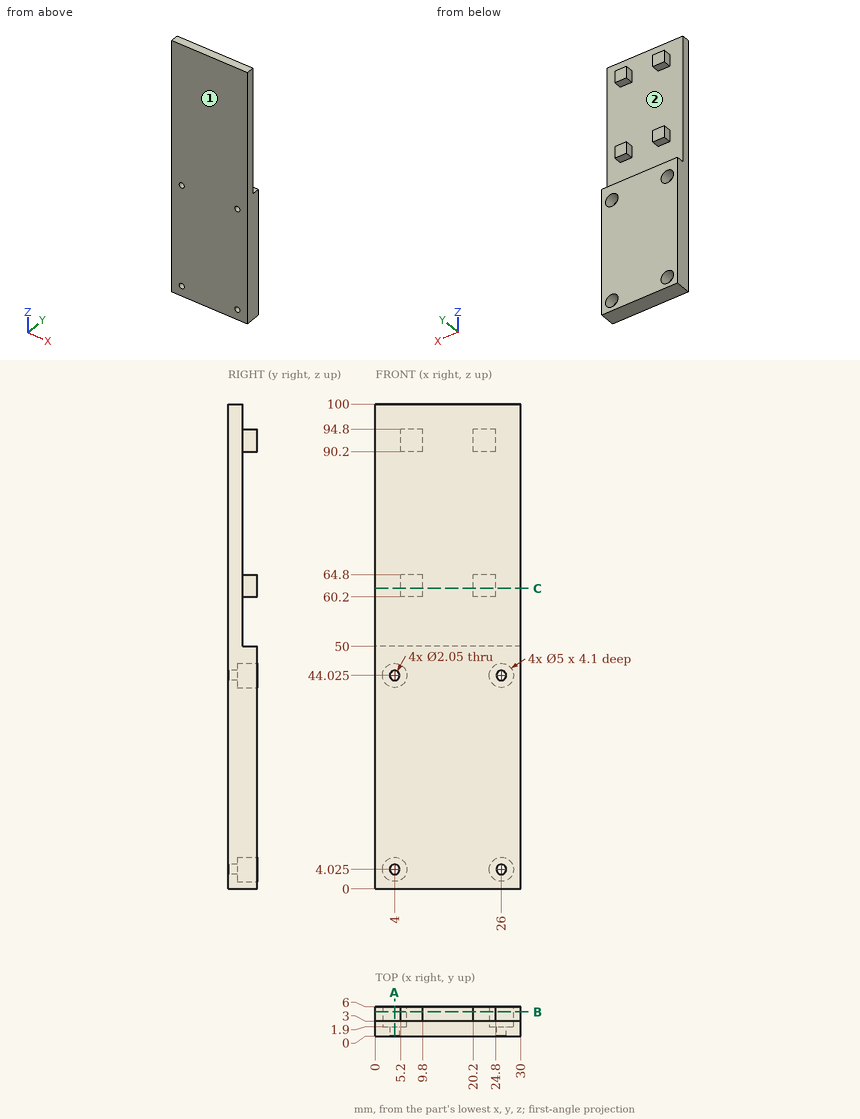
Part print with two shaded views. Sizes in mm from the minimum x, y, z corner. Give positions to 0.01 mm unless a question says otherwise; leave off trailing zeros. Order: outer loops, then holes, each group sorted by start corner. A loop starts at its lowest first (then second) coordinate and runs counter-clockwise, first axis right, second up.
1) Pin check, flat tips, straight feed: pin 1 (9 mm diameter, centred on x = 22.5, z = 74.5, fed in from +Y); pin 2 (1.5 mm diameter, centred on x = 7, y = 2.5, fed in from -Z); pin 3 (1.5 mm diameter, centred on y = 5, z = 62.5, fed in from -X); pin 4 (1.5 mm diameter, centred on x = 8.5, y = 5, fed in from +Z). Stop position of each tip, or through.
2) Mould opens along Z. For the marked faces 1 and 2 say: +Z half, -Z half, draft (parallel to the pull), parting line (faces both ways), or undercut.
3) Saw through at B-B, the plane y = 5. Count the separate pieces of the cut face and the enclosed holes in it, then the cut area to 3 significant figures.
4) Saw through at C-C, the plane z = 62. Write the cut outline in (x, y).
5) Saw through at A-A, the plane x = 4. Write the cut outline in (y, z) (3 decimals), then the cut area to 3 significant figures.
6) Wall check: probe 1 along Z at (x, y) = (4, 4.25) (3 decimals); probe 2 along Z at (x, y) = (4, 1.5); probe 3 along Y at (x, z) = (1.5, 62.5). Give the ranges that are in metal, low to high.
Computed:
1. pin 1: stops at y = 3
1. pin 2: stops at z = 0
1. pin 3: stops at x = 5.2
1. pin 4: stops at z = 94.8
2. face 1: draft
2. face 2: undercut
3. separate pieces: 5
3. enclosed holes: 4
3. area: 1,510 mm2
4. outline: (0, 0) - (30, 0) - (30, 3) - (24.8, 3) - (24.8, 6) - (20.2, 6) - (20.2, 3) - (9.8, 3) - (9.8, 6) - (5.2, 6) - (5.2, 3) - (0, 3) - close
5. outline: (0, 0) - (6, 0) - (6, 1.525) - (1.9, 1.525) - (1.9, 3) - (0, 3) - close; (0, 5.05) - (1.9, 5.05) - (1.9, 6.525) - (6, 6.525) - (6, 41.525) - (1.9, 41.525) - (1.9, 43) - (0, 43) - close; (0, 45.05) - (1.9, 45.05) - (1.9, 46.525) - (6, 46.525) - (6, 50) - (3, 50) - (3, 100) - (0, 100) - close
5. area: 401 mm2
6. probe 1: z = 0 to 1.525, 6.525 to 41.525, 46.525 to 50
6. probe 2: z = 0 to 3, 5.05 to 43, 45.05 to 100
6. probe 3: y = 0 to 3
